Can you work these out from the model? Positions are in its coordinate system, mm. A direction names the side the tool comes from. Round coordinates to 2 decimals unless told otherwise and drop trailing zeros. Write each loop counter-clockwise with the first axis right and the second up, starting at its lowest first coordinate (ties: lowest second). Pieces come first, ordered by that corner, then holes. Notation, with made-up numbers: (28, -18.5) - (84, -18.5) arc R18 ccw to (84, -10.5) - close; hole circle Ø8 at (1, 38). An arc over 180 degrees is marked (long way). One line per item, written item: value. Start each with the question number.
(1) If I drill on L1, parallel to Y at x = 0, z = -28; L2, parallel to X at y = -13, z = -3.5; L3, parallel to X at y = 1, z = -27.5, over which ranges is the centre line in solid material (lowest first)? Write a range as from..to.
(2) I want a section at B-B on z = -16. List the corners of the cut face in (x, y) for me, plus the area to 3 significant figures.
(3) Thinking about a two-plate mould opening in X: for faces 1 (the face through (7.45, 0, 2)), 2 (the face through (-9.237, -3.83, -24.93)), 3 (the face through (5.442, 9.936, -12.228)), which applies, +X half, -X half, draft (parallel to the pull), parting line (faces both ways), or undercut?
(4) I'm going to push flat-ended pins straight in: pin 1 Ø3 at (x, y) = (5.5, 14.5) entering from +Z; pin 2 Ø2 at (y, z) = (-4.5, -21) entering from +X; pin 3 Ø1.2 at (y, z) = (-1.5, 2.5) entering from +X. Where does each tip first touch, or does it pass through?
(5) On a 3-axis mill with a long thin cutter (end or side, diameter ignored), from which of +Z, -Z, +X, -X, +Y, -Y can I reach the whole of each face in a straight line? I mean faces 4 (the face through (3.673, -6.482, 1.972)), 5 (the face through (-3.673, 6.482, 1.972)), 6 (the face through (9, 0, -36)), 7 (the face through (-15.91, -12.2, -3.94)). Say none if no direction works.
(6) I want a section at A-A on z = 1. List the corners of the cut face in (x, y) for me, plus the area to 3 significant figures.
from build123d import *

# Parameters (mm, degrees)
BOSS_EXTRUDE1_DEPTH = 4
SKETCH2_R           = 10
BOSS_EXTRUDE2_DEPTH = 37
SKETCH3_R           = 1.2
CUT_EXTRUDE2_DEPTH  = 11
SKETCH6_R           = 20.05
BOSS_EXTRUDE4_DEPTH = 10
SKETCH15_R          = 21
BOSS_EXTRUDE7_DEPTH = 2
CUT_EXTRUDE4_REACH  = 49.445
SKETCH7_R           = 1.55
BOSS_EXTRUDE6_START = -5
SKETCH14_R          = 12.5
SKETCH14_R_2        = 10
BOSS_EXTRUDE6_DEPTH = 5
CUT_EXTRUDE5_REACH  = 54.058
SKETCH12_W          = 9
SKETCH12_H          = 20
SKETCH13_R          = 1.9
CUT_EXTRUDE6_DEPTH  = 9
FILLET1_R           = 10
FILLET2_R           = 2
FILLET3_R           = 2
FILLET4_R           = 2
FILLET5_R           = 2
SKETCH17_R          = 3
CUT_EXTRUDE8_DEPTH  = 10


# Some blends are built 0.0001 mm under size
with BuildPart() as part:
    # Sketch1 → Boss-Extrude1 (new body)
    with BuildSketch(Plane.XY):
        Polygon((0, 8.602519011), (-7.45, 4.301259505), (-7.45, -4.301259505), (0, -8.602519011), (7.45, -4.301259505), (7.45, 4.301259505), align=None)
    extrude(amount=BOSS_EXTRUDE1_DEPTH)

    # Sketch2 → Boss-Extrude2 (add)
    with BuildSketch(Plane(origin=(0, 0, 0), x_dir=(-1, 0, 0), z_dir=(0, 0, -1))):
        Circle(SKETCH2_R)
    extrude(amount=BOSS_EXTRUDE2_DEPTH)

    # Sketch3 → Cut-Extrude2 (cut)
    with BuildSketch(Plane(origin=(0, 0, -37), x_dir=(-1, 0, 0), z_dir=(0, 0, -1))):
        Circle(SKETCH3_R)
    extrude(amount=-CUT_EXTRUDE2_DEPTH, mode=Mode.SUBTRACT)

    # Sketch6 → Boss-Extrude4 (add)
    with BuildSketch(Plane.XY):
        Circle(SKETCH6_R)
    extrude(amount=-BOSS_EXTRUDE4_DEPTH)

    # Sketch15 → Boss-Extrude7 (add)
    with BuildSketch(Plane(origin=(0, 0, -10), x_dir=(-1, 0, 0), z_dir=(0, 0, -1))):
        Circle(SKETCH15_R)
    extrude(amount=-BOSS_EXTRUDE7_DEPTH)

    # Sketch7 → Cut-Extrude4 (cut, up to next)
    with BuildSketch(Plane.XY, mode=Mode.PRIVATE) as cut_extrude4_sk1:
        with Locations((7, 12.5)):
            Circle(SKETCH7_R)
    cut_extrude4_tool1 = extrude(cut_extrude4_sk1.sketch, amount=-CUT_EXTRUDE4_REACH, mode=Mode.PRIVATE) & part.part
    # Sketch7 → Cut-Extrude4 (cut, up to next)
    with BuildSketch(Plane.XY, mode=Mode.PRIVATE) as cut_extrude4_sk2:
        with Locations((7.325317547, -12.312177826)):
            Circle(SKETCH7_R)
    cut_extrude4_tool2 = extrude(cut_extrude4_sk2.sketch, amount=-CUT_EXTRUDE4_REACH, mode=Mode.PRIVATE) & part.part
    # Sketch7 → Cut-Extrude4 (cut, up to next)
    with BuildSketch(Plane.XY, mode=Mode.PRIVATE) as cut_extrude4_sk3:
        with Locations((-14.325317547, -0.187822174)):
            Circle(SKETCH7_R)
    cut_extrude4_tool3 = extrude(cut_extrude4_sk3.sketch, amount=-CUT_EXTRUDE4_REACH, mode=Mode.PRIVATE) & part.part
    add(cut_extrude4_tool1.solids().sort_by_distance((7, 12.5, 0))[0], mode=Mode.SUBTRACT)
    add(cut_extrude4_tool2.solids().sort_by_distance((7.325318, -12.312178, 0))[0], mode=Mode.SUBTRACT)
    add(cut_extrude4_tool3.solids().sort_by_distance((-14.325318, -0.187822, 0))[0], mode=Mode.SUBTRACT)

    # Sketch14 → Boss-Extrude6 (add)
    with BuildSketch(Plane(origin=(0, 0, -37), x_dir=(-1, 0, 0), z_dir=(0, 0, -1)).offset(BOSS_EXTRUDE6_START)):
        Circle(SKETCH14_R)
        with Locations(Location((0, 0, 0), (0, 0, 180))):
            Circle(SKETCH14_R_2, mode=Mode.SUBTRACT)
    extrude(amount=BOSS_EXTRUDE6_DEPTH)

    # Sketch12 → Cut-Extrude5 (cut, up to next)
    with BuildSketch(Plane(origin=(9, 0, 0), x_dir=(0, 0, -1), z_dir=(1, 0, 0)), mode=Mode.PRIVATE) as cut_extrude5_sk1:
        with Locations((32.5, 0)):
            Rectangle(SKETCH12_W, SKETCH12_H)
    cut_extrude5_tool1 = extrude(cut_extrude5_sk1.sketch, amount=CUT_EXTRUDE5_REACH, mode=Mode.PRIVATE) & part.part
    add(cut_extrude5_tool1.solids().sort_by_distance((9, 0, -32.5))[0], mode=Mode.SUBTRACT)

    # Sketch13 → Cut-Extrude6 (cut, symmetric)
    with BuildSketch(Plane(origin=(9, 0, 0), x_dir=(0, 0, -1), z_dir=(1, 0, 0))):
        with Locations((33, 0)):
            Circle(SKETCH13_R)
    extrude(amount=CUT_EXTRUDE6_DEPTH, both=True, mode=Mode.SUBTRACT)

    # Fillet1
    # the kernel refuses this fillet: 10 mm, written as the material it adds along each edge
    with BuildSketch(Plane(origin=(0, 0, -10), x_dir=(-1, 0, 0), z_dir=(0, 1, 0))) as fillet1_piece_1_section:
        with BuildLine():
            CenterArc((10 + FILLET1_R, -FILLET1_R), FILLET1_R, 90, 90)
            Line((10, -FILLET1_R), (10, 0))
            Line((10, 0), (10 + FILLET1_R, 0))
        make_face()
    fillet1_piece_1 = revolve(axis=Axis((0, 0, -10), (0, 0, 1)), mode=Mode.PRIVATE)
    fillet1_piece_1 = fillet1_piece_1 - Plane(origin=(7.325317547, -12.312177826, -12.841052518), x_dir=(1, 0, 0), z_dir=(0, 0, 1)) * Cylinder(1.55, 80, mode=Mode.PRIVATE)
    fillet1_piece_1 = fillet1_piece_1 - Plane(origin=(-14.325317547, -0.187822174, -12.841052518), x_dir=(1, 0, 0), z_dir=(0, 0, 1)) * Cylinder(1.55, 80, mode=Mode.PRIVATE)
    fillet1_piece_1 = fillet1_piece_1 - Plane(origin=(7, 12.5, -12.841052518), x_dir=(1, 0, 0), z_dir=(0, 0, 1)) * Cylinder(1.55, 80, mode=Mode.PRIVATE)
    add(fillet1_piece_1)

    # Fillet2
    fillet2_edges = [part.edges().sort_by_distance(p)[0] for p in [
        (21, 0, -10),
    ]]
    fillet(fillet2_edges, radius=FILLET2_R - 0.0001)  # a hair under: the kernel refuses the full size

    # Fillet3
    fillet3_edges = [part.edges().sort_by_distance(p)[0] for p in [
        (-2.236067977, 9.746794345, -32),
    ]]
    fillet(fillet3_edges, radius=FILLET3_R)

    # Fillet4
    # the kernel refuses this fillet: 2 mm, written as the material it adds along each edge
    with BuildSketch(Plane(origin=(9, 9.358898944, -28), x_dir=(1, 0, 0), z_dir=(0, -1, 0))) as fillet4_piece_1_section:
        with BuildLine():
            CenterArc((FILLET4_R, -FILLET4_R), FILLET4_R, 90, 90)
            Line((0, -FILLET4_R), (0, 0))
            Line((0, 0), (FILLET4_R, 0))
        make_face()
    fillet4_piece_1 = extrude(amount=18.717797887, mode=Mode.PRIVATE)
    fillet4_piece_1 = fillet4_piece_1 & Plane(origin=(0, 0, -28.566638375), x_dir=(-1, 0, 0), z_dir=(0, 0, 1)) * Cylinder(10, 46, mode=Mode.PRIVATE)
    add(fillet4_piece_1)

    # Fillet5
    fillet5_edges = [part.edges().sort_by_distance(p)[0] for p in [
        (-12.5, 0, -32),
    ]]
    fillet(fillet5_edges, radius=FILLET5_R)

    # Sketch17 → Cut-Extrude8 (cut)
    with BuildSketch(Plane.XY.offset(-10.5)):
        with Locations((7, 12.5)):
            Circle(SKETCH17_R)
        with Locations((7.325317547, -12.312177826)):
            Circle(SKETCH17_R)
        with Locations((-14.325317547, -0.187822174)):
            Circle(SKETCH17_R)
    extrude(amount=-CUT_EXTRUDE8_DEPTH, mode=Mode.SUBTRACT)


solid = part.part
Established:
1. L1: -10..-1.2, 1.2..10
1. L2: -15.26..5.94, 8.71..15.26
1. L3: -9.95..-0.66, 0.66..9.95
2. outline: circle Ø21.67 at (0, 0)
2. area: 369 mm2
3. face 1: +X half
3. face 2: parting line
3. face 3: undercut
4. pin 1: z = 0
4. pin 2: x = 9.37
4. pin 3: x = 7.45
5. face 4: +Z, +X, -Y
5. face 5: +Z, -X, +Y
5. face 6: -Z, +X, +Y, -Y
5. face 7: +Z
6. outline: (-7.45, -4.3) - (0, -8.6) - (7.45, -4.3) - (7.45, 4.3) - (0, 8.6) - (-7.45, 4.3) - close
6. area: 192 mm2
